Input: part model. Units: mm. Frame: model coordinates. A direction names the side the tool comes from. Give positions to 0.01 mm unless a question says otherwise; leave off trailing zeros. Loops run counter-clockwise (first coordinate to the right, second up) from the corner with the lowest first, then second, coordinate; pieces in that order, holes last. Notation, with made-up numbers: M 2.5,-3 L 54.5,-3 A35 ccw 54.5,36 Z; hole C 38,37 d8. An arc over 180 degrees is marked long. Answer as a JSON object with one key per item and string values. Group by question number.
1) Draft query along Y for faces 4 (the flat face through (4, 0, 18)), 5 (the flat face through (12, 282, 31)), 6 (the flat face through (9, 9, 18)), 7 (the flat face through (13, 544, 17)). Return one class per face: +Y half, -Y half, draft (parallel to the pull), parting line (faces both ways), or undercut.
2) Ray query, L1, parallel to Z at x = 1.5, y = 322; L2, parallel to Y at x = 12.5, z = 27.5. Return the intervals inside material, ascending.
3) First-contact query: P1, Ø5.5, axis at y = 11, z = 12.5, coming from the +X side; P2, Ø4.5, axis at x = 13.5, z = 15.5, coming from the -Y side; P3, Ø10, axis at x = 14.5, z = 30.5, coming from the +Y side. Flat tips, straight axial feed; report the tip coordinate or a pass-through.
4) Section query D-D on y = 253. Return loops of the section in (x, z), plus the area to 3 significant figures.
5) Access query for faces 1 (the flat face through (9, 277, 0)), 2 (the flat face through (13, 18, 17)), 3 (the flat face through (9, 553, 18)). Directions: +Z, -Z, +X, -X, +Y, -Y. A direction counts if a zero-diameter tool reaches every point of the face in a straight line with its end or side. Return the directions, or none.
6) Section query A-A on x = 3. Return loops of the section in (y, z), plus the area to 3 significant figures.
7) Section query B-B on z = 14. Return loops of the section in (x, y).
8) Section query C-C on y = 94.5. Return loops of the section in (x, z).
from build123d import *

# Parameters (mm, degrees)
F1_DEPTH = 18
F0_W     = 18
F0_H     = 31
F0_H_2   = 4
F2_DEPTH = 9
F0_W_2   = 213
F3_DEPTH = 14


with BuildPart() as f1:
    # F0 (on Right) → F1 (new body)
    with BuildSketch(Plane.YZ):
        Polygon((18, 31), (18, 0), (544, 0), (544, 31), (331, 31), (281, 31), (231, 31), align=None)
    extrude(amount=F1_DEPTH)

    # F0 (on Right) → F2 (join)
    with BuildSketch(Plane.YZ):
        with Locations((9, 15.5)):
            Rectangle(F0_W, F0_H)
        with Locations((553, 15.5)):
            Rectangle(F0_W, F0_H)
        with Locations((9, 33)):
            Rectangle(F0_W, F0_H_2)
        with Locations((553, 33)):
            Rectangle(F0_W, F0_H_2)
    extrude(amount=F2_DEPTH)

    # F0 (on Right) → F3 (join)
    with BuildSketch(Plane.YZ):
        with Locations((124.5, 33)):
            Rectangle(F0_W_2, F0_H_2)
        with Locations((437.5, 33)):
            Rectangle(F0_W_2, F0_H_2)
    extrude(amount=F3_DEPTH)


solid = f1.part
Output:
{
 "1": {"face 4": "-Y half", "face 5": "undercut", "face 6": "draft", "face 7": "+Y half"},
 "2": {"L1": "z = 0 to 31", "L2": "y = 18 to 544"},
 "3": {"P1": "stops at x = 9", "P2": "stops at y = 18", "P3": "stops at y = 544"},
 "4": {"outline": "M 0,0 L 18,0 L 18,31 L 0,31 Z", "area": "558 mm^2"},
 "5": {"face 1": "-Z, +X, -X, +Y, -Y", "face 2": "+Z, -Z, +X, -Y", "face 3": "+Z, -Z, +X, +Y"},
 "6": {"outline": "M 0,0 L 562,0 L 562,35 L 331,35 L 331,31 L 231,31 L 231,35 L 0,35 Z", "area": "19,300 mm^2"},
 "7": {"outline": "M 0,0 L 9,0 L 9,18 L 18,18 L 18,544 L 9,544 L 9,562 L 0,562 Z"},
 "8": {"outline": "M 0,0 L 18,0 L 18,31 L 14,31 L 14,35 L 0,35 Z"}
}
